from build123d import *

# Parameters (mm, degrees)
SKETCH1_R           = 127
BOSS_EXTRUDE1_DEPTH = 12.7
CUT_EXTRUDE1_DEPTH  = 6.35
SKETCH2_3_R         = 9.525
CUT_EXTRUDE2_DEPTH  = 13.7


with BuildPart() as part:
    # Sketch1 → Boss-Extrude1 (new body)
    with BuildSketch(Plane(origin=(0, 0, 0), x_dir=(1, 0, 0), z_dir=(0, 1, 0))):
        Circle(SKETCH1_R)
    extrude(amount=BOSS_EXTRUDE1_DEPTH)

    # Sketch2 → Cut-Extrude1 (cut)
    with BuildSketch(Plane(origin=(0, 12.7, 0), x_dir=(1, 0, 0), z_dir=(0, 1, 0))):
        with BuildLine():
            Line((-31.430896424, 31.430896424), (-76.332177029, 76.332177029))
            ThreePointArc((-76.332177029, 76.332177029), (-89.757144648, 59.973806654), (-99.732795535, 41.310676524))
            Line((-99.732795535, 41.310676524), (-41.06644522, 17.010278569))
            ThreePointArc((-41.06644522, 17.010278569), (-36.958824267, 24.695096858), (-31.430896424, 31.430896424))
        make_face()
        with BuildLine():
            Line((-44.45, 0), (-107.95, 0))
            ThreePointArc((-107.95, 0), (-105.87577102, -21.060000262), (-99.732795535, -41.310676524))
            Line((-99.732795535, -41.310676524), (-41.06644522, -17.010278569))
            ThreePointArc((-41.06644522, -17.010278569), (-43.595905714, -8.671764814), (-44.45, 0))
        make_face()
        with BuildLine():
            Line((-31.430896424, -31.430896424), (-76.332177029, -76.332177029))
            ThreePointArc((-76.332177029, -76.332177029), (-59.973806654, -89.757144648), (-41.310676524, -99.732795535))
            Line((-41.310676524, -99.732795535), (-17.010278569, -41.06644522))
            ThreePointArc((-17.010278569, -41.06644522), (-24.695096858, -36.958824267), (-31.430896424, -31.430896424))
        make_face()
        with BuildLine():
            Line((0, -44.45), (0, -107.95))
            ThreePointArc((0, -107.95), (21.060000262, -105.87577102), (41.310676524, -99.732795535))
            Line((41.310676524, -99.732795535), (17.010278569, -41.06644522))
            ThreePointArc((17.010278569, -41.06644522), (8.671764814, -43.595905714), (0, -44.45))
        make_face()
        with BuildLine():
            Line((31.430896424, -31.430896424), (76.332177029, -76.332177029))
            ThreePointArc((76.332177029, -76.332177029), (89.757144648, -59.973806654), (99.732795535, -41.310676524))
            Line((99.732795535, -41.310676524), (41.06644522, -17.010278569))
            ThreePointArc((41.06644522, -17.010278569), (36.958824267, -24.695096858), (31.430896424, -31.430896424))
        make_face()
        with BuildLine():
            ThreePointArc((44.45, 0), (43.595905714, 8.671764814), (41.06644522, 17.010278569))
            Line((41.06644522, 17.010278569), (99.732795535, 41.310676524))
            ThreePointArc((99.732795535, 41.310676524), (105.87577102, 21.060000262), (107.95, 0))
            Line((107.95, 0), (44.45, 0))
        make_face()
        with BuildLine():
            Line((31.430896424, 31.430896424), (76.332177029, 76.332177029))
            ThreePointArc((76.332177029, 76.332177029), (59.973806654, 89.757144648), (41.310676524, 99.732795535))
            Line((41.310676524, 99.732795535), (17.010278569, 41.06644522))
            ThreePointArc((17.010278569, 41.06644522), (24.695096858, 36.958824267), (31.430896424, 31.430896424))
        make_face()
        with BuildLine():
            Line((0, 44.45), (0, 107.95))
            ThreePointArc((0, 107.95), (-21.060000262, 105.87577102), (-41.310676524, 99.732795535))
            Line((-41.310676524, 99.732795535), (-17.010278569, 41.06644522))
            ThreePointArc((-17.010278569, 41.06644522), (-8.671764814, 43.595905714), (0, 44.45))
        make_face()
    extrude(amount=-CUT_EXTRUDE1_DEPTH, mode=Mode.SUBTRACT)

    # Sketch2_3 → Cut-Extrude2 (cut, through all)
    with BuildSketch(Plane(origin=(0, 12.7, 0), x_dir=(1, 0, 0), z_dir=(0, 1, 0))):
        with Locations((0, 127)):
            Circle(SKETCH2_3_R)
        with Locations((127, 0)):
            Circle(SKETCH2_3_R)
        with Locations((0, -127)):
            Circle(SKETCH2_3_R)
        with Locations((-127, 0)):
            Circle(SKETCH2_3_R)
        with BuildLine():
            Line((10.992753262, -5.08), (-10.992753262, -5.08))
            ThreePointArc((-10.992753262, -5.08), (-28.575, 0), (-10.992753262, 5.08))
            Line((-10.992753262, 5.08), (10.992753262, 5.08))
            ThreePointArc((10.992753262, 5.08), (28.575, 0), (10.992753262, -5.08))
        make_face()
    extrude(amount=-CUT_EXTRUDE2_DEPTH, mode=Mode.SUBTRACT)


solid = part.part
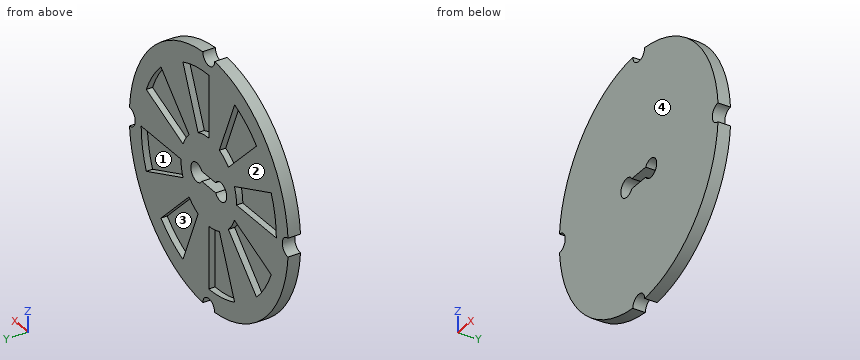
Read the model definition and answer for the solid it produces. Units are mm, in the model's axes. Face numbers are marked on the shaded views. A direction names the side the tool comes from. Round coordinates to 2 decimals unless told otherwise and drop trailing zeros. Loops run counter-clockwise (first coordinate to the right, second up) from the corner with the lowest first, then second, coordinate; pieces in that order, holes last.
Q1. Section B-B on z = -38 is taken. Write down the section's boundary in (x, y).
Q2. Section C-C on x = 82.5 is taken. Write down the section's boundary in (y, z).
Q3. Consider probe 1 along X at (y, z) = (2.5, 0) (3 decimals); probe 2 along X at (y, z) = (11, -96.5); probe 3 along Z at (x, y) = (19.05, 6.5) (3 decimals). Determine where each line is inside the solid, lowest interval first.
Q4. Which of the six approach directions +Z, -Z, +X, -X, +Y, -Y give full straight-line access (tool end or side, diameter ignored) to the marked faces 1 and 2?
Q5. Determine the mould class of the marked faces 3 and 4 for opening direction Z: released by +Z, released by -Z, zero draft, split by the parting line, or undercut.
Q6. Section A-A on x = -24 is taken. Write down the section's boundary in (y, z).
Q7. Each of these flat-tipped pins is pushed along its axis until it touches: pin 1 (1.9 mm diameter, centred on y = 8.5, z = -84, fed in from -X); pin 2 (20.5 mm diameter, centred on x = -80.5, z = 30.5, fed in from +Y); pin 3 (3 mm diameter, centred on x = -83.5, y = 10, fed in from +Z); pin 4 (7 mm diameter, centred on x = 71, y = 10, fed in from -Z). Where does it stop, or does it pass through?
Q8. Section D-D on z = 80.5 is taken. Write down the section's boundary in (x, y), and give its area (3 significant figures).
Output:
1. outline: (-121.18, 0) - (121.18, 0) - (121.18, 12.7) - (101.04, 12.7) - (101.04, 6.35) - (91.74, 6.35) - (91.74, 12.7) - (38, 12.7) - (38, 6.35) - (23.06, 6.35) - (23.06, 12.7) - (-38, 12.7) - (-38, 6.35) - (-91.74, 6.35) - (-91.74, 12.7) - (-121.18, 12.7) - close
2. outline: (0, -96.55) - (12.7, -96.55) - (12.7, -34.17) - (6.35, -34.17) - (6.35, 0) - (12.7, 0) - (12.7, 34.17) - (6.35, 34.17) - (6.35, 69.62) - (12.7, 69.62) - (12.7, 96.55) - (0, 96.55) - close
3. probe 1: x = -117.475 to -28.575, 28.575 to 117.475
3. probe 2: x = -82.56 to -39.97, 0 to 39.97, 48.38 to 82.56
3. probe 3: z = -125.563 to -45.991, -40.161 to -9.525, 9.525 to 45.991, 106.256 to 125.563
4. face 1: +Y
4. face 2: +Z, -Z, +X, -X, +Y
5. face 3: undercut
5. face 4: zero draft
6. outline: (0, -124.71) - (12.7, -124.71) - (12.7, -105.25) - (6.35, -105.25) - (6.35, -57.94) - (12.7, -57.94) - (12.7, -8.14) - (0, -8.14) - close; (0, 8.14) - (12.7, 8.14) - (12.7, 37.41) - (6.35, 37.41) - (6.35, 57.94) - (12.7, 57.94) - (12.7, 124.71) - (0, 124.71) - close
7. pin 1: stops at x = -96.08
7. pin 2: stops at y = 12.7
7. pin 3: stops at z = 96.98
7. pin 4: stops at z = -107.58
8. outline: (-98.23, 0) - (98.23, 0) - (98.23, 12.7) - (33.34, 12.7) - (33.34, 6.35) - (0, 6.35) - (0, 12.7) - (-33.34, 12.7) - (-33.34, 6.35) - (-71.92, 6.35) - (-71.92, 12.7) - (-98.23, 12.7) - close
8. area: 2,040 mm2
